Part model, mm, in its own coordinate system. A direction names the side the tool comes from. Round coordinates to 2 decimals unless told otherwise and drop trailing zeros. Loops run counter-clockwise (first coordinate to the right, second up) from the corner with the lowest first, then second, coordinate; pieces in that order, holes last. Notation, with made-up numbers: M -1.5,-18.5 L 16.5,-18.5 A35 ccw 16.5,19.5 Z; hole C 84,58.5 d4. An arc over 180 degrees is marked long. Write each question's results on one line, items separated by ' | '.
from build123d import *

# Parameters (mm, degrees)
SKETCH2_W                      = 27
SKETCH2_H                      = 25
SKETCH2_W_2                    = 3
BOSS_EXTRUDE1_DEPTH            = 3
SKETCH2_3_W                    = 3
SKETCH2_3_H                    = 25
BOSS_EXTRUDE2_DEPTH            = 20
BOSS_EXTRUDE3_START            = 20
SKETCH2_4_W                    = 20
SKETCH2_4_H                    = 25
BOSS_EXTRUDE3_DEPTH            = 3
BOSS_EXTRUDE4_START            = 12.5
SKETCH3_W                      = 27
SKETCH3_H                      = 28
BOSS_EXTRUDE4_DEPTH            = 3
CBORE_FOR_M4_SHCS1_D           = 4.5
CBORE_FOR_M4_SHCS1_DEPTH       = 10
CBORE_FOR_M4_SHCS1_CBORE_D     = 4.502
CBORE_FOR_M4_SHCS1_CBORE_DEPTH = 4
CBORE_FOR_M4_SHCS1_TIP         = 1.351936393
CBORE_FOR_M4_SHCS2_D           = 4.5
CBORE_FOR_M4_SHCS2_DEPTH       = 10
CBORE_FOR_M4_SHCS2_CBORE_D     = 4.503
CBORE_FOR_M4_SHCS2_CBORE_DEPTH = 4
CBORE_FOR_M4_SHCS2_TIP         = 1.351936393
CHAMFER1_SIZE                  = 1


with BuildPart() as part:
    # Sketch2 → Boss-Extrude1 (new body)
    with BuildSketch(Plane.XY):
        with Locations((-26.5, 0)):
            Rectangle(SKETCH2_W, SKETCH2_H)
        with Locations((26.5, 0)):
            Rectangle(SKETCH2_W, SKETCH2_H)
        with Locations((-11.5, 0)):
            Rectangle(SKETCH2_W_2, SKETCH2_H)
        with Locations((11.5, 0)):
            Rectangle(SKETCH2_W_2, SKETCH2_H)
    extrude(amount=-BOSS_EXTRUDE1_DEPTH)

    # Sketch2<3> → Boss-Extrude2 (add)
    with BuildSketch(Plane.XY):
        with Locations((-11.5, 0)):
            Rectangle(SKETCH2_3_W, SKETCH2_3_H)
        with Locations((11.5, 0)):
            Rectangle(SKETCH2_3_W, SKETCH2_3_H)
    extrude(amount=BOSS_EXTRUDE2_DEPTH)

    # Sketch2<4> → Boss-Extrude3 (add)
    with BuildSketch(Plane.XY.offset(BOSS_EXTRUDE3_START)):
        Rectangle(SKETCH2_4_W, SKETCH2_4_H)
    extrude(amount=-BOSS_EXTRUDE3_DEPTH)

    # Sketch3 → Boss-Extrude4 (add)
    with BuildSketch(Plane(origin=(0, 0, 0), x_dir=(1, 0, 0), z_dir=(0, 1, 0)).offset(BOSS_EXTRUDE4_START)):
        with Locations((-26.5, 14)):
            Rectangle(SKETCH3_W, SKETCH3_H)
        Polygon((-13, 28), (-13, 0), (-10, 0), (-10, 3), (-10, 28), align=None)
        Polygon((-10, 0), (-13, 0), (-13, -20), (13, -20), (13, 0), (10, 0), (10, -17), (-10, -17), align=None)
        with Locations((26.5, 14)):
            Rectangle(SKETCH3_W, SKETCH3_H)
        Polygon((10, 0), (13, 0), (13, 28), (10, 28), (10, 3), align=None)
    extrude(amount=BOSS_EXTRUDE4_DEPTH)

    # Sketch6 → CBORE for M5 Hex Head Cap Screw1 (revolve, cut)
    with BuildSketch(Plane(origin=(0, 0, 20), x_dir=(0, -1, 0), z_dir=(1, 0, 0))):
        Polygon((0, 0), (0, 4.652366702), (2.75, 3), (2.75, 3.65), (2.7505, 0), align=None)
    revolve(axis=Axis((0, 0, 26.35), (0, 0, -1)), mode=Mode.SUBTRACT)

    # CBORE for M4 SHCS1
    with Locations(Plane.XY):
        with Locations((30, 0), (-30, 0)):
            CounterBoreHole(CBORE_FOR_M4_SHCS1_D / 2, CBORE_FOR_M4_SHCS1_CBORE_D / 2, CBORE_FOR_M4_SHCS1_CBORE_DEPTH, depth=CBORE_FOR_M4_SHCS1_DEPTH)
            with Locations((0, 0, -(CBORE_FOR_M4_SHCS1_DEPTH + CBORE_FOR_M4_SHCS1_TIP / 2))):  # 118° drill point
                Cone(0, CBORE_FOR_M4_SHCS1_D / 2, CBORE_FOR_M4_SHCS1_TIP, mode=Mode.SUBTRACT)

    # CBORE for M4 SHCS2
    with Locations(Plane(origin=(0, 15.5, 0), x_dir=(1, 0, 0), z_dir=(0, 1, 0))):
        with Locations((30, 14), (-30, 14)):
            CounterBoreHole(CBORE_FOR_M4_SHCS2_D / 2, CBORE_FOR_M4_SHCS2_CBORE_D / 2, CBORE_FOR_M4_SHCS2_CBORE_DEPTH, depth=CBORE_FOR_M4_SHCS2_DEPTH)
            with Locations((0, 0, -(CBORE_FOR_M4_SHCS2_DEPTH + CBORE_FOR_M4_SHCS2_TIP / 2))):  # 118° drill point
                Cone(0, CBORE_FOR_M4_SHCS2_D / 2, CBORE_FOR_M4_SHCS2_TIP, mode=Mode.SUBTRACT)

    # Chamfer1
    chamfer1_edges = [part.edges().sort_by_distance(p)[0] for p in [
        (-10, 0, -3),
        (-26.5, -12.5, 0),
        (-13, 1.5, 0),
        (0, -12.5, 20),
        (-13, -12.5, 10),
        (-13, 1.5, 20),
        (-40, 0, -3),
        (0, -12.5, 17),
        (13, 1.5, 0),
        (40, 1.5, 0),
        (26.5, -12.5, 0),
        (40, -12.5, -1.5),
        (10, -12.5, 7),
        (10, 0, -3),
        (40, 0, -3),
        (25, -12.5, -3),
        (13, 1.5, 20),
        (13, -12.5, 10),
        (-25, -12.5, -3),
        (-13, 15.5, 10),
        (40, 12.5, -15.5),
        (25, 12.5, -28),
        (-40, 1.5, 0),
        (40, 14, -28),
        (10, 12.5, -15.5),
        (10, 14, -28),
        (-10, 15.5, -5.5),
        (-25, 15.5, -28),
        (-10, 14, -28),
        (-40, 15.5, -14),
        (-40, 14, -28),
        (-26.5, 15.5, 0),
        (0, 15.5, 20),
        (13, 15.5, 10),
        (26.5, 15.5, 0),
        (40, 15.5, -14),
        (25, 15.5, -28),
        (10, 15.5, -5.5),
        (0, 15.5, 17),
        (-40, 12.5, -15.5),
        (-25, 12.5, -28),
        (-10, 12.5, -15.5),
        (-40, -12.5, -1.5),
        (-10, -12.5, 7),
    ]]
    chamfer(chamfer1_edges, length=CHAMFER1_SIZE)


solid = part.part
Item 1: Band-saw the part on C-C on z = -14. Give the cut face in (x, y).
Filled sheet:
outline: M -40,13.5 L -39,12.5 L -32.25,12.5 L -32.25,15.5 L -39,15.5 L -40,14.5 Z; M -27.75,12.5 L -11,12.5 L -10,13.5 L -10,14.5 L -11,15.5 L -27.75,15.5 Z; M 10,13.5 L 11,12.5 L 27.75,12.5 L 27.75,15.5 L 11,15.5 L 10,14.5 Z; M 32.25,12.5 L 39,12.5 L 40,13.5 L 40,14.5 L 39,15.5 L 32.25,15.5 Z
Item 2: Drop flat-ended pins along their axis: P1, Ø7.5, axis at x = -21.5, y = 3.5, coming from the +Z side; P2, Ø9, axis at y = 0, z = 11.5, coming from the -X side; P3, Ø4, axis at x = -26, y = -1.5, coming from the -Z side; P4, Ø12, axis at y = -1, z = -11, coming from the +X side. Give the stop position or say it passes through.
Filled sheet:
P1: z = 0 | P2: x = -13 | P3: z = -3 | P4: through
Item 3: Band-saw the part on A-A on z = -19.5. Give the cut face in (x, y).
Filled sheet:
outline: M -40,13.5 L -39,12.5 L -11,12.5 L -10,13.5 L -10,14.5 L -11,15.5 L -39,15.5 L -40,14.5 Z; M 10,13.5 L 11,12.5 L 39,12.5 L 40,13.5 L 40,14.5 L 39,15.5 L 11,15.5 L 10,14.5 Z
Item 4: Which spindle directions (+Z, -Z, +X, -X, +Y, -Y) get a long thin tool onto all of the face, cutting with end or side? Do faces 1 (the flat face through (-13, 1, 10)), 2 (the flat face through (26, 1, 0)), 3 (the flat face through (-0.2, -12.5, 18.7)), 4 (the flat face through (25, 1, -3)). Say none if no direction does.
Filled sheet:
face 1: +Z, -X, +Y, -Y | face 2: +Z, +X, +Y, -Y | face 3: +Z, -Z, +X, -X, -Y | face 4: -Z, +X, -X, -Y
Item 5: Band-saw the part on D-D on y = -9.5. Give the cut face in (x, z), and give its area (3 significant figures).
Filled sheet:
outline: M -40,-2 L -39,-3 L -11,-3 L -10,-2 L -10,17 L 10,17 L 10,-2 L 11,-3 L 39,-3 L 40,-2 L 40,-1 L 39,0 L 14,0 L 13,1 L 13,19 L 12,20 L -12,20 L -13,19 L -13,1 L -14,0 L -39,0 L -40,-1 Z | area: 357 mm^2
Item 6: Band-saw the part on B-B on x = 30. Give the cut face in (y, z), and give its area (3 significant figures).
Filled sheet:
outline: M -12.5,-2 L -11.5,-3 L -2.25,-3 L -2.25,0 L -11.5,0 L -12.5,-1 Z; M 2.25,-3 L 12.5,-3 L 12.5,-11.75 L 15.5,-11.75 L 15.5,-1 L 14.5,0 L 2.25,0 Z; M 12.5,-27 L 13.5,-28 L 14.5,-28 L 15.5,-27 L 15.5,-16.25 L 12.5,-16.25 Z | area: 129 mm^2
Item 7: Two-plate mould, pull along Z, no slides. Class faces 5 (the flat face through (13.2, 15.1, 0.2)), 6 (the flat face through (-10, 1, 10)), 7 (the cylindrical face through (31.21, 14.02, -15.9)): +Z half, -Z half, draft (parallel to the pull), parting line (faces both ways), or undercut.
Filled sheet:
face 5: +Z half | face 6: draft | face 7: undercut
Item 8: Wall check: L1, parallel to Y at x = 0, z = 18; L2, parallel to X at y = 11.75, z = 3; L3, parallel to Z at x = -30, y = 13.6. Give the ranges that are in metal, low to high.
Filled sheet:
L1: -12.5 to -2.75, 2.75 to 15.5 | L2: -13 to -10, 10 to 13 | L3: -28 to -16.25, -11.75 to 0
